The figure shows three views and two pictorial views of one solid part (mm, origin at its lowest corner). Answer the questions. Round coordinates to 2 decimals unless told otherwise and drop trailing zeros. Write each loop counter-clockwise with the first axis right and the second up, starting at its lowest first coordinate (ties: lowest second). Pieces come first, ordered by that corner, then holes.
Item 1: Find section A-A on z = 30. Give the vertices of the cut face in (x, y), then the cut area to 3 significant figures.
Item 2: Find section B-B on y = 20.75. Give the vertices of the cut face in (x, z), then the cut area to 3 significant figures.
Item 3: Each of these flat-tipped pins is pushed along its axis until it touches: pin 1 (1 mm diameter, centred on y = 5, z = 11, fed in from -X); pin 2 (10 mm diameter, centred on x = 245.5, y = 3, fed in from +Z); pin 3 (8 mm diameter, centred on y = 19, z = 30, fed in from +X). Where does it stop, or does it pass through?
Item 4: Find section C-C on z = 6.5. Give the vertices of the cut face in (x, y), then the cut area to 3 significant figures.
Item 5: Find the intervals of material crossed by probe 1 along X at (y, z) = (21.25, 31.5); probe 2 along Z at (x, y) = (220, 15.75); probe 3 along X at (y, z) = (23.5, 24), in increasing order.
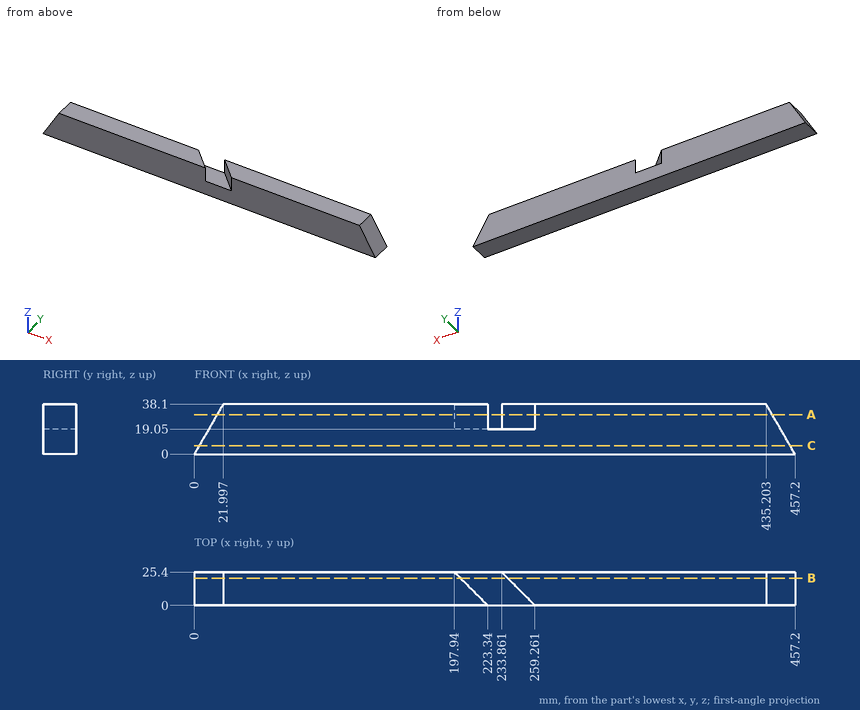
Check values:
1. outline: (17.32, 0) - (223.34, 0) - (197.94, 25.4) - (17.32, 25.4) - close; (233.86, 25.4) - (259.26, 0) - (439.88, 0) - (439.88, 25.4) - close
1. area: 9,820 mm2
2. outline: (0, 0) - (457.2, 0) - (435.2, 38.1) - (238.51, 38.1) - (238.51, 19.05) - (202.59, 19.05) - (202.59, 38.1) - (22, 38.1) - close
2. area: 15,900 mm2
3. pin 1: stops at x = 6.06
3. pin 2: stops at z = 19.05
3. pin 3: stops at x = 442.19
4. outline: (3.75, 0) - (453.45, 0) - (453.45, 25.4) - (3.75, 25.4) - close
4. area: 11,400 mm2
5. probe 1: x = 18.19 to 202.09, 238.01 to 439.01
5. probe 2: z = 0 to 19.05
5. probe 3: x = 13.86 to 199.84, 235.76 to 443.34
